Study the drawing (mm; zero at the part's minimum x, y, z) and answer. Give positions to 0.01 mm unless a question says otherwise; leave off trailing zeros. Order: outer loops, then holes, each group sorted by start corner. A loop starts at its lowest first (then second) coordinate and runs counter-clockwise, first axis right, second up.
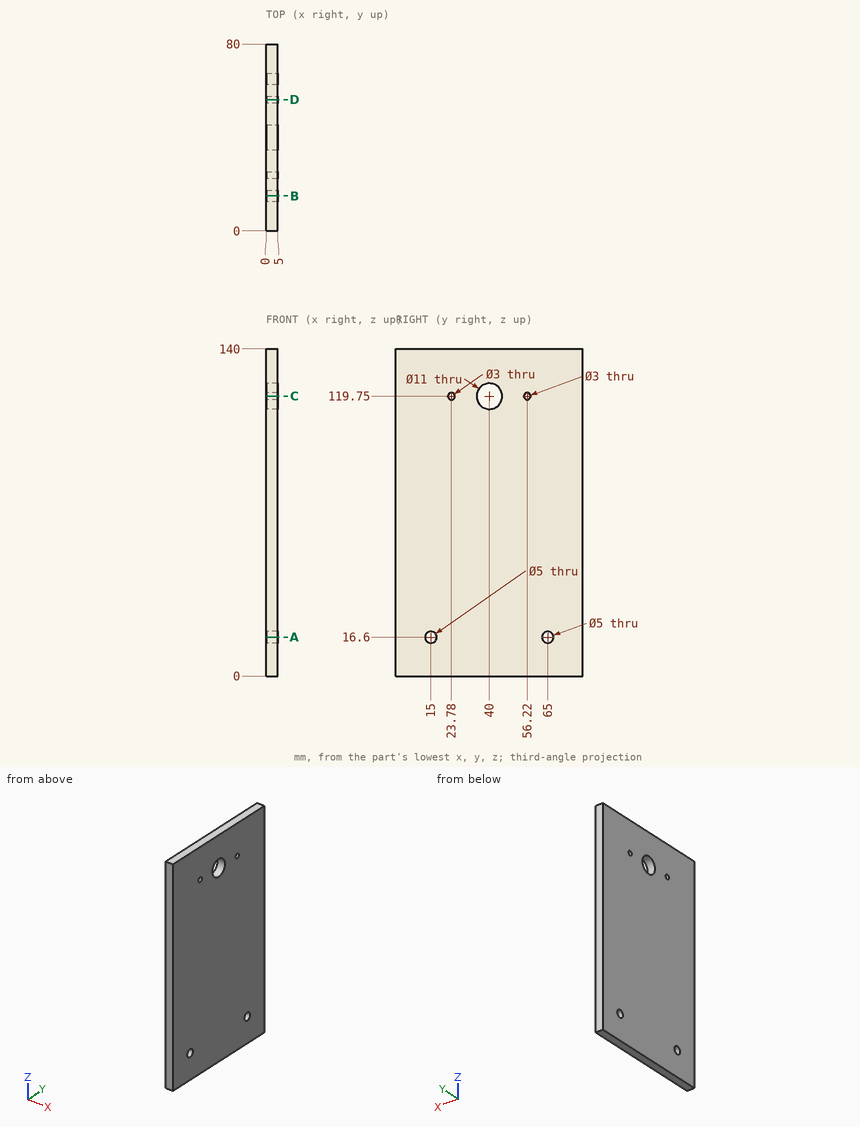
1) Straight lines are drawn through the part: probe 1 along Z at (x, y) = (1.65, 15); probe 2 along Z at (x, y) = (3.1, 56.22); probe 3 along Y at (x, z) = (0.55, 116.5). For each, find the intervals that lie inside material, in ascending order.
Geometry says:
probe 1: z = 0 to 14.1, 19.1 to 140
probe 2: z = 0 to 118.25, 121.25 to 140
probe 3: y = 0 to 35.56, 44.44 to 80
2) Find section C-C (z = 119.75). Write down the section's boundary in (x, y), then the cut area to 3 significant figures.
Geometry says:
outline: (0, 0) - (5, 0) - (5, 22.28) - (0, 22.28) - close; (0, 25.28) - (5, 25.28) - (5, 34.5) - (0, 34.5) - close; (0, 45.5) - (5, 45.5) - (5, 54.72) - (0, 54.72) - close; (0, 57.72) - (5, 57.72) - (5, 80) - (0, 80) - close
area: 315 mm2
3) Find section A-A (z = 16.6). Write down the section's boundary in (x, y), then the cut area to 3 significant figures.
Geometry says:
outline: (0, 0) - (5, 0) - (5, 12.5) - (0, 12.5) - close; (0, 17.5) - (5, 17.5) - (5, 62.5) - (0, 62.5) - close; (0, 67.5) - (5, 67.5) - (5, 80) - (0, 80) - close
area: 350 mm2
4) Given P1, Ø1.8, axis at y = 23.78, z = 119.75, coming from the -X side; P2, Ø1.5, axis at x = 1.5, z = 94.5, coming from the -Y side, each flat-ended and moving along its own axis, determine where each tip first touches the part or whether it passes through.
Geometry says:
P1: passes through
P2: stops at y = 0
5) Find section B-B (y = 15). Write down the section's boundary in (x, z).
Geometry says:
outline: (0, 0) - (5, 0) - (5, 14.1) - (0, 14.1) - close; (0, 19.1) - (5, 19.1) - (5, 140) - (0, 140) - close
6) Find section D-D (y = 56.22). Write down the section's boundary in (x, z), then the cut area to 3 significant figures.
Geometry says:
outline: (0, 0) - (5, 0) - (5, 118.25) - (0, 118.25) - close; (0, 121.25) - (5, 121.25) - (5, 140) - (0, 140) - close
area: 685 mm2
